Source: CAD feature listing. Evaluate the final solid. Frame: model axes, mm. Face numbers are marked on the shaded views. A direction names the side the tool comes from. Give positions to 0.01 mm unless a question says otherwise; leave off trailing zeros. Loops run counter-clockwise (first coordinate to the right, second up) from the corner with the lowest first, then second, coordinate; pieces in that order, holes last. Notation, with made-up numbers: M -19,5.5 L 31,5.5 A14 ccw 31,18.5 Z; hole C 86.25,-21.75 d11. An arc over 180 degrees is marked long. Put each result on its own line as item: value. Start each with the question number.
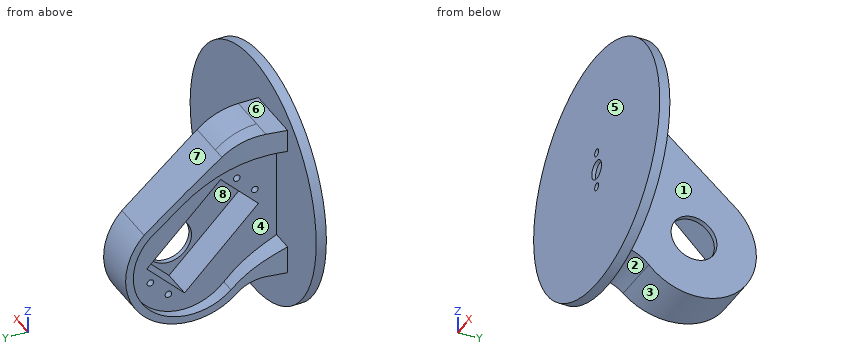
```python
from build123d import *

# Parameters (mm, degrees)
SKETCH2_R                       = 48.5
BOSS_EXTRUDE1_DEPTH             = 4
SKETCH4_R                       = 1.5
CUT_EXTRUDE2_DEPTH              = 69.705894944
SKETCH5_R                       = 3.75
CUT_EXTRUDE3_DEPTH              = 1.5
BOSS_EXTRUDE2_DEPTH             = 14
CUT_EXTRUDE5_REACH              = 97.597
SKETCH9_R                       = 1.3
CUT_EXTRUDE6_DEPTH              = 7.5
CUT_EXTRUDE9_REACH              = 96.471
SKETCH11_R                      = 9
BOSS_EXTRUDE7_DEPTH             = 9
BOSS_EXTRUDE7_DIRECTION_2_REACH = 104.912
BOSS_EXTRUDE10_DEPTH            = 9
CUT_EXTRUDE17_DEPTH             = 95.342420983
CUT_EXTRUDE17_DEPTH_BACK        = 95.342420983


with BuildPart() as part:
    # Sketch2 → Boss-Extrude1 (new body)
    with BuildSketch(Plane(origin=(0, 0, 0), x_dir=(1, 0, 0), z_dir=(0, 1, 0))):
        with Locations(Location((0, 0, 0), (0, 0, 270))):
            Circle(SKETCH2_R)
    extrude(amount=BOSS_EXTRUDE1_DEPTH)

    # Sketch4 → Cut-Extrude2 (cut, through all)
    with BuildSketch(Plane.XZ):
        with Locations(Location((0, 7.25, 0), (0, 0, 270))):
            Circle(SKETCH4_R)
        with Locations(Location((0, -7.25, 0), (0, 0, 270))):
            Circle(SKETCH4_R)
    extrude(amount=-CUT_EXTRUDE2_DEPTH, mode=Mode.SUBTRACT)

    # Sketch5 → Cut-Extrude3 (cut)
    with BuildSketch(Plane.XZ):
        with Locations(Location((0, 0, 0), (0, 0, 270))):
            Circle(SKETCH5_R)
    extrude(amount=-CUT_EXTRUDE3_DEPTH, mode=Mode.SUBTRACT)

    # Sketch7 → Boss-Extrude2 (add)
    with BuildSketch(Plane(origin=(-4, 0, 0), x_dir=(0, 0, -1), z_dir=(1, 0, 0))):
        with BuildLine():
            Line((23.129947874, 4), (23.129947874, 11.644549616))
            ThreePointArc((23.129947874, 11.644549616), (24.589048403, 18.743749901), (28.729797284, 24.692011643))
            ThreePointArc((28.729797284, 24.692011643), (29.313383054, 55.284736897), (-1.284289494, 55.479275971))
            Line((-1.284289494, 55.479275971), (-27.227315747, 29.536249718))
            ThreePointArc((-27.227315747, 29.536249718), (-32.64663453, 21.425665997), (-34.549646217, 11.858580188))
            Line((-34.549646217, 11.858580188), (-34.549646217, 4))
            Line((-34.549646217, 4), (23.129947874, 4))
        make_face()
    extrude(amount=-BOSS_EXTRUDE2_DEPTH)

    # Sketch8 → Cut-Extrude5 (cut, up to next)
    with BuildSketch(Plane(origin=(-6, 0, 0), x_dir=(0, 0, -1), z_dir=(1, 0, 0)), mode=Mode.PRIVATE) as cut_extrude5_sk1:
        Polygon((-15.249648422, 25.957567857), (13.741729607, 54.948945886), (28.590972012, 40.099703481), (-0.400406017, 11.108325452), align=None)
    cut_extrude5_tool1 = extrude(cut_extrude5_sk1.sketch, amount=-CUT_EXTRUDE5_REACH, mode=Mode.PRIVATE) & part.part
    add(cut_extrude5_tool1.solids().sort_by_distance((-6, 33.028636, -6.670662))[0], mode=Mode.SUBTRACT)

    # Sketch9 → Cut-Extrude6 (cut)
    with BuildSketch(Plane.ZY.offset(18)):
        with Locations((-20.105690637, 53.534732323)):
            Circle(SKETCH9_R)
        with Locations((-27.176758449, 46.463664511)):
            Circle(SKETCH9_R)
        with Locations((6.764367048, 12.522539014)):
            Circle(SKETCH9_R)
        with Locations((13.83543486, 19.593606826)):
            Circle(SKETCH9_R)
    extrude(amount=-CUT_EXTRUDE6_DEPTH, mode=Mode.SUBTRACT)

    # Sketch11 → Cut-Extrude9 (cut, up to next)
    with BuildSketch(Plane(origin=(-4, 0, 0), x_dir=(0, 0, -1), z_dir=(1, 0, 0)), mode=Mode.PRIVATE) as cut_extrude9_sk1:
        with Locations((13.918506302, 40.276480176)):
            Circle(SKETCH11_R)
    cut_extrude9_tool1 = extrude(cut_extrude9_sk1.sketch, amount=-CUT_EXTRUDE9_REACH, mode=Mode.PRIVATE) & part.part
    add(cut_extrude9_tool1.solids().sort_by_distance((-4, 40.27648, -13.918506))[0], mode=Mode.SUBTRACT)

    # Sketch17 → Boss-Extrude7 (add)
    with BuildSketch(Plane.ZY.offset(18)):
        with BuildLine():
            ThreePointArc((34.549646217, 11.858580188), (33.008342843, 20.500891953), (28.574482006, 28.077569775))
            ThreePointArc((28.574482006, 28.077569775), (27.915386359, 28.820289685), (27.227315747, 29.536249718))
            Line((27.227315747, 29.536249718), (1.284289494, 55.479275971))
            Line((1.284289494, 55.479275971), (26.295003593, 26.127182305))
            ThreePointArc((26.295003593, 26.127182305), (30.194232218, 19.461281607), (31.549646217, 11.858580188))
            Line((31.549646217, 11.858580188), (31.549646217, 4))
            Line((31.549646217, 4), (34.549646217, 4))
            Line((34.549646217, 4), (34.549646217, 11.858580188))
        make_face()
        with BuildLine():
            Line((28.574482006, 28.077569775), (3.405609837, 57.600596315))
            ThreePointArc((3.405609837, 57.600596315), (-31.461505391, 57.378912253), (-30.796489049, 22.517434639))
            ThreePointArc((-30.796489049, 22.517434639), (-27.345864981, 17.560549854), (-26.129947874, 11.644549616))
            Line((-26.129947874, 11.644549616), (-26.129947874, 4))
            Line((-26.129947874, 4), (-23.129947874, 4))
            Line((-23.129947874, 4), (-23.129947874, 11.644549616))
            ThreePointArc((-23.129947874, 11.644549616), (-24.589048403, 18.743749901), (-28.729797284, 24.692011643))
            ThreePointArc((-28.729797284, 24.692011643), (-29.313383054, 55.284736897), (1.284289494, 55.479275971))
            Line((1.284289494, 55.479275971), (27.227315747, 29.536249718))
            ThreePointArc((27.227315747, 29.536249718), (27.915386359, 28.820289685), (28.574482006, 28.077569775))
        make_face()
    extrude(amount=BOSS_EXTRUDE7_DEPTH)

    # Boss-Extrude7 direction 2: up to this face of the body (flat: up to its plane)
    boss_extrude7_direction_2_end = Plane(part.part.faces().sort_by_distance((-4, 28.276431801, -1.649713195))[0])
    # Sketch17 → Boss-Extrude7 direction 2 (add, up to the picked face)
    with BuildSketch(Plane.ZY.offset(18), mode=Mode.PRIVATE) as boss_extrude7_direction_2_sk1:
        with BuildLine():
            ThreePointArc((34.549646217, 11.858580188), (33.008342843, 20.500891953), (28.574482006, 28.077569775))
            ThreePointArc((28.574482006, 28.077569775), (27.915386359, 28.820289685), (27.227315747, 29.536249718))
            Line((27.227315747, 29.536249718), (1.284289494, 55.479275971))
            Line((1.284289494, 55.479275971), (26.295003593, 26.127182305))
            ThreePointArc((26.295003593, 26.127182305), (30.194232218, 19.461281607), (31.549646217, 11.858580188))
            Line((31.549646217, 11.858580188), (31.549646217, 4))
            Line((31.549646217, 4), (34.549646217, 4))
            Line((34.549646217, 4), (34.549646217, 11.858580188))
        make_face()
    boss_extrude7_direction_2_tool1 = split(extrude(boss_extrude7_direction_2_sk1.sketch, amount=-BOSS_EXTRUDE7_DIRECTION_2_REACH, mode=Mode.PRIVATE), bisect_by=boss_extrude7_direction_2_end, keep=Keep.BOTH, mode=Mode.PRIVATE)
    # Sketch17 → Boss-Extrude7 direction 2 (add, up to the picked face)
    with BuildSketch(Plane.ZY.offset(18), mode=Mode.PRIVATE) as boss_extrude7_direction_2_sk2:
        with BuildLine():
            Line((28.574482006, 28.077569775), (3.405609837, 57.600596315))
            ThreePointArc((3.405609837, 57.600596315), (-31.461505391, 57.378912253), (-30.796489049, 22.517434639))
            ThreePointArc((-30.796489049, 22.517434639), (-27.345864981, 17.560549854), (-26.129947874, 11.644549616))
            Line((-26.129947874, 11.644549616), (-26.129947874, 4))
            Line((-26.129947874, 4), (-23.129947874, 4))
            Line((-23.129947874, 4), (-23.129947874, 11.644549616))
            ThreePointArc((-23.129947874, 11.644549616), (-24.589048403, 18.743749901), (-28.729797284, 24.692011643))
            ThreePointArc((-28.729797284, 24.692011643), (-29.313383054, 55.284736897), (1.284289494, 55.479275971))
            Line((1.284289494, 55.479275971), (27.227315747, 29.536249718))
            ThreePointArc((27.227315747, 29.536249718), (27.915386359, 28.820289685), (28.574482006, 28.077569775))
        make_face()
    boss_extrude7_direction_2_tool2 = split(extrude(boss_extrude7_direction_2_sk2.sketch, amount=-BOSS_EXTRUDE7_DIRECTION_2_REACH, mode=Mode.PRIVATE), bisect_by=boss_extrude7_direction_2_end, keep=Keep.BOTH, mode=Mode.PRIVATE)
    add(boss_extrude7_direction_2_tool1.solids().sort_by(Axis((-18, 4.612919, 33.049646), (1, 0, 0)))[0])
    add(boss_extrude7_direction_2_tool2.solids().sort_by(Axis((-18, 43.147366, 14.895406), (1, 0, 0)))[0])

    # Sketch25 → Boss-Extrude10 (add)
    with BuildSketch(Plane.ZY.offset(18)):
        with BuildLine():
            ThreePointArc((-28.729797284, 24.692011643), (-24.589048403, 18.743749901), (-23.129947874, 11.644549616))
            Line((-23.129947874, 11.644549616), (-23.129947874, 4))
            Line((-23.129947874, 4), (-15.129947874, 4))
            add(Edge.make_bspline(
                [(-28.729797284, 24.692011643), (-21.954867515, 18.253200081), (-19.09405247, 12.798017691), (-15.129947874, 4)],
                knots=[0, 0, 0, 0, 1, 1, 1, 1], degree=3))
        make_face()
        with BuildLine():
            add(Edge.make_bspline(
                [(11.751619577, 43.19501844), (26.551255916, 25.8264495), (25.549646217, 4)],
                knots=[0, 0, 0, 1, 1, 1], degree=2))
            Line((25.549646217, 4), (31.549646217, 4))
            Line((31.549646217, 4), (31.549646217, 11.858580188))
            ThreePointArc((31.549646217, 11.858580188), (30.194232218, 19.461281607), (26.295003593, 26.127182305))
            Line((26.295003593, 26.127182305), (11.751619577, 43.19501844))
        make_face()
    extrude(amount=BOSS_EXTRUDE10_DEPTH)

    # Sketch29 → Cut-Extrude17 (cut, two sides: drawn at the far end of the back side and taken through both)
    with BuildSketch(Plane.XY.offset(-CUT_EXTRUDE17_DEPTH_BACK)):
        with BuildLine():
            Line((-21, 64.776480176), (-27, 64.776480176))
            Line((-27, 64.776480176), (-27, 4))
            Line((-27, 4), (-26.5, 4))
            add(Edge.make_bspline(
                [(-21, 64.776480176), (-21.220459696, 34.140901434), (-26.5, 4)],
                knots=[0, 0, 0, 1, 1, 1], degree=2))
        make_face()
    extrude(amount=CUT_EXTRUDE17_DEPTH + CUT_EXTRUDE17_DEPTH_BACK, mode=Mode.SUBTRACT)


solid = part.part
```
1. Section B-B, the plane z = -7.25. State how many separate pieces and enclosed holes the cut face has, plus the area to 3 significant figures.
2. Contact query for flat-ended pins moving along their axis: pin 1 (2 mm diameter, centred on y = 46.46, z = -27.18, fed in from +X); pin 2 (4 mm diameter, centred on x = 0, z = -7.25, fed in from +Y); pin 3 (3.5 mm diameter, centred on y = 19.59, z = 13.84, fed in from -X); pin 4 (16 mm diameter, centred on y = 40.28, z = -13.92, fed in from -X). Output: stop coordinate, or through.
3. Section A-A, the plane x = 0. Output: boundary loops of the cut face in (y, z).
4. Section C-C, the plane x = 42. Output: boundary loops of the cut face in (y, z).
5. Ray query, line 1 (X direction, y = 1, z = 0); line 2 (X direction, y = 9, z = -5); line 3 (Y direction, x = 29, z = -14). Return the intervals inside material, ascending.
6. Pull-direction query (Y, two-part tool) for the marked faces 5, 6, 7 and 8; classes: released by +Y, released by -Y, zero draft, split by the parting line, or undercut.
7. Set-up query: the marked faces 1, 2, 3 and 4. Return all of +Z, -Z, +X, -X, +Y, -Y with unobstructed straight access to the full face (end or side cutting, diameter ignored); none if empty.
Results found:
1. separate pieces: 3
1. enclosed holes: 0
1. area: 838 mm²
2. pin 1: x = -4
2. pin 2: y = 4
2. pin 3: x = -18
2. pin 4: through
3. outline: M 0,-48.5 L 4,-48.5 L 4,-8.75 L 0,-8.75 Z; M 0,-5.75 L 4,-5.75 L 4,5.75 L 0,5.75 L 0,3.75 L 1.5,3.75 L 1.5,-3.75 L 0,-3.75 Z; M 0,8.75 L 4,8.75 L 4,48.5 L 0,48.5 Z
4. outline: M 0,-24.25 L 4,-24.25 L 4,24.25 L 0,24.25 Z
5. line 1: -48.5 to -3.75, 3.75 to 48.5
5. line 2: -18 to -4
5. line 3: 0 to 4
6. face 5: released by -Y
6. face 6: zero draft
6. face 7: released by +Y
6. face 8: undercut
7. face 1: +Z, -Z, +X, +Y
7. face 2: -Z, +X, -X
7. face 3: +X, -X
7. face 4: -X
